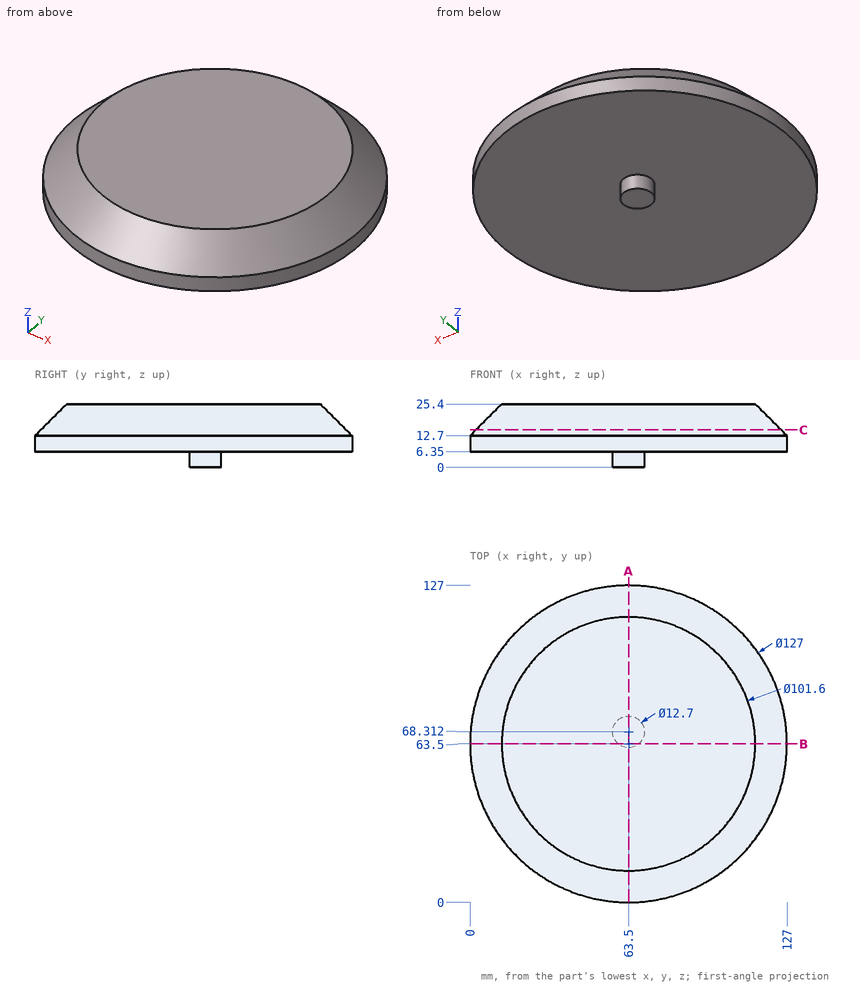
Design review of the part shown in the three views and the two pictorial views. Dimensions are in mm from the part's minimum x, y and z. Round coordinates to 2 decimals unless told otherwise and drop trailing zeros. Loops run counter-clockwise (first coordinate to the right, second up) from the corner with the lowest first, then second, coordinate; pieces in that order, holes last.
1) Consider section B-B on y = 63.5. State the section outline as (x, z) points, then the cut area to 3 significant figures.
Values follow:
outline: (0, 6.35) - (59.36, 6.35) - (59.36, 0) - (67.64, 0) - (67.64, 6.35) - (127, 6.35) - (127, 12.7) - (114.3, 25.4) - (12.7, 25.4) - (0, 12.7) - close
area: 2,310 mm2
2) Wall thickness on line 1 along Z through (x, y) = (87.5, 43.5); line 2 along Y through (x, z) = (21.5, 23) (1 decimal); line 3 along X through (y, z) = (18, 8.75) (1 decimal): over which ranges is each line inside the solid? List them lowest first.
Values follow:
line 1: z = 6.35 to 25.4
line 2: y = 30.8 to 96.2
line 3: x = 19.2 to 107.8
3) Consider section C-C on z = 15. State the section outline as (x, y) points, then the cut area to 3 significant figures.
Values follow:
outline: circle Ø122.4 at (63.5, 63.5)
area: 11,800 mm2
4) Clearance check with flat-ended pins moving along their axes: P1, Ø5, axis at x = 19.5, z = 13, coming from the +Y side; P2, Ø6, axis at y = 19, z = 7, coming from the +X side; P3, Ø8, axis at y = 72, z = 22.5, coming from the -X side; P4, Ø6, axis at x = 87.5, y = 15.5, coming from the +Z side. State where each tip first meets the part, or that it passes through.
Values follow:
P1: stops at y = 111.55
P2: stops at x = 111.56
P3: stops at x = 6.39
P4: stops at z = 25.4
5) Consider section A-A on x = 63.5. State the section outline as (y, z) points.
Values follow:
outline: (0, 6.35) - (61.96, 6.35) - (61.96, 0) - (74.66, 0) - (74.66, 6.35) - (127, 6.35) - (127, 12.7) - (114.3, 25.4) - (12.7, 25.4) - (0, 12.7) - close
